Design review of the part built by this model. Coordinates are the model's own, in mm. A direction names the side the tool comes from. Coordinates: 2 decimals unless noted, no trailing zeros. Order: outer loops, then holes, each group sorted by start corner. A loop starts at its lowest first (then second) coordinate and runs counter-clockwise, first axis right, second up. Notation, with made-up numbers: M -39.75,65 L 13.25,65 A10 cw 13.25,80 Z; hole C 78,-22.5 d9. An arc over 180 degrees is marked long. Answer in a Markdown table with one row per item.
Autodesk Inventor part; units mm, degrees
ref_plane "YZ Plane" through (0, 0, 0) normal (1, 0, 0) x (0, 1, 0)
ref_plane "XZ Plane" through (0, 0, 0) normal (0, 1, 0) x (-1, 0, 0)
ref_plane "XY Plane" through (0, 0, 0) normal (0, 0, 1) x (1, 0, 0)
sketch "ｽｹｯﾁ1" plane through (0, 0, 0) normal (0, 0, 1) x (1, 0, 0)
  line L0 (-1.8494, 20) -> (18.1506, 20)
  line L1 (18.1506, 20) -> (18.1506, 12)
  line L2 (18.1506, 12) -> (-1.8494, 12)
  line L3 (-1.8494, 12) -> (-1.8494, 20)
  line L4 (-1.8494, 20) -> (6.1506, 20)
  line L5 (6.1506, 20) -> (6.1506, -25)
  line L6 (1.1506, -30) -> (-1.8494, -30)
  line L7 (-1.8494, -30) -> (-1.8494, 20)
  line L8 (6.1506, -25) -> (1.1506, -30)
  point P0 (6.1506, -30)
  dimension "d0" = 20
  dimension "d1" = 8
  dimension "d2" = 50
  dimension "d3" = 5
  dimension "d4" = 5
  dimension "d5" = 8
extrude "Extrusion1" add sketch "ｽｹｯﾁ1" along normal blind 20
properties part number "Robot-Clamp"
(1) Add section B-B, the plane x = 11. Give the boundary of the cut face in (y, z).
Return value:
| item | result |
|---|---|
| outline | M 12,0 L 20,0 L 20,20 L 12,20 Z |
(2) Insertion check: pin 1 Ø3.5 at (x, z) = (10.5, 9.5) entering from -Y; pin 2 Ø8 at (y, z) = (-4.5, 13.5) entering from +X; pin 3 Ø1.5 at (x, z) = (6.5, 6) entering from -Y. Each pin has a flat end and moves straight along its axis. Give the tip position at first contact, or say it passes through.
Return value:
| item | result |
|---|---|
| pin 1 | stops at y = 12 |
| pin 2 | stops at x = 6.15 |
| pin 3 | stops at y = -25.4 |
(3) For line 1 along Y through (x, z) = (12, 9.5); line 2 along X through (y, z) = (-14, 1); line 3 along Y through (x, z) = (1.75, 15.25), list the stretches that pass through material, from the lowest coordinate up. Write a range as from..to.
Return value:
| item | result |
|---|---|
| line 1 | y = 12..20 |
| line 2 | x = -1.85..6.15 |
| line 3 | y = -29.4..20 |
(4) Add section C-C, the plane y = -7. Give the boundary of the cut face in (x, z), and give its area (3 significant figures).
Return value:
| item | result |
|---|---|
| outline | M -1.85,0 L 6.15,0 L 6.15,20 L -1.85,20 Z |
| area | 160 mm2 |
(5) Add section A-A, the plane z = 17.25. Give the boundary of the cut face in (x, y), and give its area (4 significant figures).
Return value:
| item | result |
|---|---|
| outline | M -1.85,-30 L 1.15,-30 L 6.15,-25 L 6.15,12 L 18.15,12 L 18.15,20 L -1.85,20 Z |
| area | 483.5 mm2 |
(6) For faces 1 (the flat face through (6.151, -6, 10)), 2 (the flat face through (4, 1, 20)), list the 3-axis set-ups (+Z, -Z, +X, -X, +Y, -Y) from which the entire face can be reached by the end or side of a thin tool; tool diameter is ignored.
Return value:
| item | result |
|---|---|
| face 1 | +Z, -Z, +X, -Y |
| face 2 | +Z, +X, -X, +Y, -Y |
